Geometry: final body of the model. Coordinates: model frame, mm. A direction names the side the tool comes from. Coordinates: 2 decimals unless noted, no trailing zeros. Write each loop counter-clockwise with the first axis right and the second up, starting at its lowest first coordinate (ties: lowest second). Pieces come first, ordered by that corner, then holes.
from build123d import *

# Parameters (mm, degrees)
SKETCH1_W           = 15
SKETCH1_H           = 35
BOSS_EXTRUDE1_DEPTH = 32
SKETCH4_W           = 15
SKETCH4_H           = 23
CUT_EXTRUDE2_DEPTH  = 16.5
SKETCH7_R           = 2.5
BOSS_EXTRUDE2_DEPTH = 3
SKETCH9_W           = 50
SKETCH9_H           = 40
BOSS_EXTRUDE3_DEPTH = 5
SKETCH10_W          = 7
SKETCH10_H          = 4.5
CUT_EXTRUDE3_DEPTH  = 10


with BuildPart() as part:
    # Sketch1 → Boss-Extrude1 (new body)
    with BuildSketch(Plane.XY):
        Rectangle(SKETCH1_W, SKETCH1_H)
    extrude(amount=BOSS_EXTRUDE1_DEPTH)

    # Sketch4 → Cut-Extrude2 (cut)
    with BuildSketch(Plane.XY.offset(32)):
        with Locations((0, -1.5)):
            Rectangle(SKETCH4_W, SKETCH4_H)
    extrude(amount=-CUT_EXTRUDE2_DEPTH, mode=Mode.SUBTRACT)

    # Sketch7 → Boss-Extrude2 (add)
    with BuildSketch(Plane(origin=(0, 0, 0), x_dir=(-1, 0, 0), z_dir=(0, 0, -1))):
        with Locations((0, -6.4)):
            Circle(SKETCH7_R)
    extrude(amount=BOSS_EXTRUDE2_DEPTH)

    # Sketch9 → Boss-Extrude3 (add)
    with BuildSketch(Plane(origin=(0, 17.5, 0), x_dir=(1, 0, 0), z_dir=(0, 1, 0))):
        with Locations((0, -20)):
            Rectangle(SKETCH9_W, SKETCH9_H)
    extrude(amount=BOSS_EXTRUDE3_DEPTH)

    # Sketch10 → Cut-Extrude3 (cut)
    with BuildSketch(Plane.ZY.offset(7.5)):
        with Locations((19, -15.25)):
            Rectangle(SKETCH10_W, SKETCH10_H)
    extrude(amount=-CUT_EXTRUDE3_DEPTH, mode=Mode.SUBTRACT)


solid = part.part
Item 1: Pin query (flat end, axial travel): pin 1 (8 mm diameter, centred on x = -2, y = 13, fed in from +Z); pin 2 (4 mm diameter, centred on y = 11.5, z = 9.5, fed in from -X); pin 3 (1 mm diameter, centred on x = 18.5, z = 17.5, fed in from -Y). Return the tip coordinate at first contact, or that it passes through.
Derived:
pin 1: stops at z = 32
pin 2: stops at x = -7.5
pin 3: stops at y = 17.5
Item 2: Pull-direction query (Y, two-part tool) for faces 6 (the flat face through (0, 10, 24)), 7 (the flat face through (0, -15, 32)), 8 (the flat face through (2, -13, 26)), 9 (the cylindrical face through (2, -7.9, -1.5)); classes: released by +Y, released by -Y, zero draft, split by the parting line, or undercut.
Derived:
face 6: undercut
face 7: zero draft
face 8: undercut
face 9: split by the parting line
Item 3: Section B-B, the plane z = 27. Output: boundary loops of the cut face in (x, y), plus the area to 3 significant figures.
Derived:
outline: (-25, 17.5) - (-7.5, 17.5) - (-7.5, 10) - (7.5, 10) - (7.5, 17.5) - (25, 17.5) - (25, 22.5) - (-25, 22.5) - close; (-7.5, -17.5) - (7.5, -17.5) - (7.5, -13) - (-7.5, -13) - close
area: 430 mm2
Item 4: Section D-D, the plane z = 9. Output: boundary loops of the cut face in (x, y).
Derived:
outline: (-25, 17.5) - (-7.5, 17.5) - (-7.5, -17.5) - (7.5, -17.5) - (7.5, 17.5) - (25, 17.5) - (25, 22.5) - (-25, 22.5) - close
Item 5: Section C-C, the plane y = -6.4. Output: boundary loops of the cut face in (x, z).
Derived:
outline: (-7.5, 0) - (-2.5, 0) - (-2.5, -3) - (2.5, -3) - (2.5, 0) - (7.5, 0) - (7.5, 15.5) - (-7.5, 15.5) - close
Item 6: Section A-A, the plane x = 0. Output: boundary loops of the cut face in (y, z).
Derived:
outline: (-17.5, 0) - (-8.9, 0) - (-8.9, -3) - (-3.9, -3) - (-3.9, 0) - (22.5, 0) - (22.5, 40) - (17.5, 40) - (17.5, 32) - (10, 32) - (10, 15.5) - (-17.5, 15.5) - close; (-17.5, 22.5) - (-13, 22.5) - (-13, 32) - (-17.5, 32) - close
Item 7: Set-up query: faces 1 (the flat face through (7.5, 0, 12)), 2 (the flat face through (0, 22.5, 20)), 3 (the flat face through (2.5, -15, 19)), 4 (the flat face through (-7.5, 4, 9)), 5 (the flat face through (0, 14, 32)). Return all of +Z, -Z, +X, -X, +Y, -Y with unobstructed straight access to the full face (end or side cutting, diameter ignored); none if empty.
Derived:
face 1: +Z, -Z, +X, -Y
face 2: +Z, -Z, +X, -X, +Y
face 3: -X, -Y
face 4: +Z, -Z, -X, -Y
face 5: +Z, +X, -X, -Y
Item 8: Material intervals for probe 1 along Y at (x, z) = (0.5, 29.5); probe 2 along X at (y, z) = (-15, 5.5); probe 3 along Y at (x, z) = (-12.5, 36), sorted ascending.
Derived:
probe 1: y = -17.5 to -13, 10 to 22.5
probe 2: x = -7.5 to 7.5
probe 3: y = 17.5 to 22.5
